Here's how the part is built. I have some questions about the finished solid (model axes, mm). A direction names the side the tool comes from. Give positions to 0.01 mm unless a question says otherwise; leave off trailing zeros. Loops run counter-clockwise (first coordinate to the right, second up) from the corner with the lowest first, then second, coordinate; pieces in that order, holes last. Notation, with made-up numbers: (27, 82.5) - (84, 82.5) arc R29 ccw to (84, 109.5) - close; hole circle Ø3 at (37.25, 85). An arc over 180 degrees is marked (long way). One line per item, written item: value. Start each with the question number.
```python
from build123d import *

# Parameters (mm, degrees)
BOSS_EXTRUDE1_DEPTH = 5
SKETCH2_R           = 2.5
CUT_EXTRUDE1_DEPTH  = 31.618621785


with BuildPart() as part:
    # Sketch1 → Boss-Extrude1 (new body)
    with BuildSketch(Plane.XY):
        Polygon((-7.5, 27.5), (-7.5, 17.5), (7.5, 17.5), (7.5, 27.5), (12.5, 27.5), (12.5, -27.5), (-12.5, -27.5), (-12.5, 27.5), align=None)
    extrude(amount=BOSS_EXTRUDE1_DEPTH)

    # Sketch2 → Cut-Extrude1 (cut, through all)
    with BuildSketch(Plane.XY.offset(5)):
        with Locations((0, -17.5)):
            Circle(SKETCH2_R)
    extrude(amount=-CUT_EXTRUDE1_DEPTH, mode=Mode.SUBTRACT)


solid = part.part
```
(1) Will this pin go through, and if not, where does the flat tip stop? pin 1 (4 mm diameter, centred on x = 0, y = -17.5, fed in from +Z).
(2) Please list where these lines run through material, in increasing order: probe 1 along Y at (x, z) = (0, 1.75); probe 2 along X at (y, z) = (19, 2.6); probe 3 along Y at (x, z) = (-3, 3.85). Write a range as from..to.
(3) For faces 5 (the face through (0, 17.5, 2)), 6 (the face through (12.5, 0, 2)), which set-ups out of +Z, -Z, +X, -X, +Y, -Y let a thin tool reach every point of the face, with its end or its side?
(4) If we section it at A-A on y = -17.5: List the corners of the cut face in (x, z) for me.
(5) If we mould it in two halves opening along Y, with no side actions, what happens to faces 1 (the face through (-0.54, -19.94, 2.54)), 2 (the face through (10, 27.5, 2)), 3 (the face through (-7.5, 23, 2)), 4 (the face through (0, -27.5, 2))? For each: pulls with the +Y half, pulls with the -Y half, needs draft (parallel to the pull), parting line crosses it, or undercut.
(6) If we section it at C-C on z = 3.5: List the corners of the cut face in (x, y) for me, plus the area to 3 significant figures.
(7) If we section it at B-B on x = 0: List the corners of the cut face in (y, z) for me, plus the area to 3 significant figures.
Found:
1. pin 1: through
2. probe 1: -27.5..-20, -15..17.5
2. probe 2: -12.5..-7.5, 7.5..12.5
2. probe 3: -27.5..17.5
3. face 5: +Z, -Z, +Y
3. face 6: +Z, -Z, +X, +Y, -Y
4. outline: (-12.5, 0) - (-2.5, 0) - (-2.5, 5) - (-12.5, 5) - close; (2.5, 0) - (12.5, 0) - (12.5, 5) - (2.5, 5) - close
5. face 1: undercut
5. face 2: pulls with the +Y half
5. face 3: needs draft
5. face 4: pulls with the -Y half
6. outline: (-12.5, -27.5) - (12.5, -27.5) - (12.5, 27.5) - (7.5, 27.5) - (7.5, 17.5) - (-7.5, 17.5) - (-7.5, 27.5) - (-12.5, 27.5) - close; hole circle Ø5 at (0, -17.5)
6. area: 1,210 mm^2
7. outline: (-27.5, 0) - (-20, 0) - (-20, 5) - (-27.5, 5) - close; (-15, 0) - (17.5, 0) - (17.5, 5) - (-15, 5) - close
7. area: 200 mm^2
